```python
from build123d import *

# Parameters (mm, degrees)
F1_DEPTH    = 34.29
F2_T1_DEPTH = 186.4119082094
F2_T4_ANGLE = 180
F4_DEPTH    = 50.8
F6_DEPTH    = 27.94


# Not quite as in the source:
# - a fillet or chamfer that OpenCascade refuses, or shapes differently, is made with other operations: its cross-section is extruded or revolved along the edge and cut away or added


with BuildPart() as f1:
    # F0 (on Top) → F1 (new body)
    with BuildSketch(Plane.XY):
        with BuildLine():
            ThreePointArc((-39.772413671, 45.8196774125), (0, 6.0472637415), (39.772413671, 45.8196774125))
            Line((39.772413671, 45.8196774125), (-39.772413671, 45.8196774125))
        make_face()
        with BuildLine():
            Line((-39.772413671, 45.8196774125), (39.772413671, 45.8196774125))
            ThreePointArc((39.772413671, 45.8196774125), (0, 85.5920910835), (-39.772413671, 45.8196774125))
        make_face()
        with BuildLine():
            Line((39.772413671, -45.8196774125), (39.772413671, 45.8196774125))
            ThreePointArc((39.772413671, 45.8196774125), (0, 6.0472637415), (-39.772413671, 45.8196774125))
            Line((-39.772413671, 45.8196774125), (-39.772413671, -45.8196774125))
            Line((-39.772413671, -45.8196774125), (39.772413671, -45.8196774125))
        make_face()
    extrude(amount=F1_DEPTH)

    # F2: fillet of radius 38.1 on 3 edges, made by hand

    # F2_s2 → F2_t1 (cut)
    with BuildSketch(Plane.XZ.offset(-45.8196774125)):
        with BuildLine():
            ThreePointArc((-39.772413671, 0), (-27.4216493001, 24.4457162358), (-1.8633923173, 34.29))
            Line((-1.8633923173, 34.29), (-39.772413671, 34.29))
            Line((-39.772413671, 34.29), (-39.772413671, 0))
        make_face()
        with BuildLine():
            ThreePointArc((39.772413671, 0), (27.4216493001, 24.4457162358), (1.8633923173, 34.29))
            Line((1.8633923173, 34.29), (39.772413671, 34.29))
            Line((39.772413671, 34.29), (39.772413671, 0))
        make_face()
    extrude(amount=F2_T1_DEPTH, mode=Mode.SUBTRACT)

    # F2_s3 → F2_t4 (revolve, cut)
    with BuildSketch(Plane.XZ.offset(-45.8196774125)):
        with BuildLine():
            ThreePointArc((39.772413671, 0), (27.4216493001, 24.4457162358), (1.8633923173, 34.29))
            Line((1.8633923173, 34.29), (39.772413671, 34.29))
            Line((39.772413671, 34.29), (39.772413671, 0))
        make_face()
    revolve(axis=Axis((0, 45.8196774125, 34.29), (0, 0, 1)), revolution_arc=F2_T4_ANGLE, mode=Mode.SUBTRACT)

    # F3 (on Right) → F4 (cut)
    with BuildSketch(Plane.YZ):
        with BuildLine():
            add(Edge.make_bspline(
                [(26.3266563416, 13.0248842761), (26.3266563416, -3.7878693164), (55.981522426, 4.6185074799), (85.6363885105, 13.0248842761), (55.981522426, 21.4312610723), (26.3266563416, 29.8376378686), (26.3266563416, 13.0248842761)],
                knots=[0, 0, 0, 2.0943951024, 2.0943951024, 4.1887902048, 4.1887902048, 6.2831853072, 6.2831853072, 6.2831853072], degree=2, weights=[1, 0.5, 1, 0.5, 1, 0.5, 1]))
        make_face()
    extrude(amount=F4_DEPTH, mode=Mode.SUBTRACT)

    # F5 (on Right) → F6 (join)
    with BuildSketch(Plane.YZ):
        with BuildLine():
            add(Edge.make_bspline(
                [(65.8664852381, 13.2574718446), (65.8664852381, 30.580146327), (34.8160881549, 21.9188090858), (3.7656910717, 13.2574718446), (34.8160881549, 4.5961346033), (65.8664852381, -4.0652026379), (65.8664852381, 13.2574718446)],
                knots=[0, 0, 0, 2.0943951024, 2.0943951024, 4.1887902048, 4.1887902048, 6.2831853072, 6.2831853072, 6.2831853072], degree=2, weights=[1, 0.5, 1, 0.5, 1, 0.5, 1]))
        make_face()
    extrude(amount=F6_DEPTH)


solid = f1.part
```
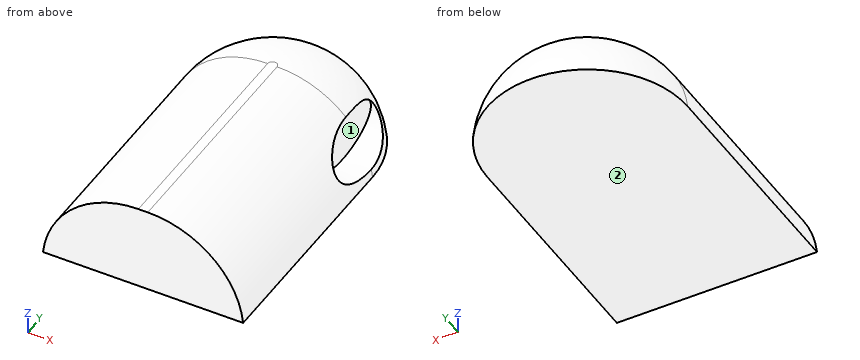
Check sheet for the modelled part. Datum: model origin and axes. Units: mm. Face numbers are marked on the shaded views. A direction names the side the tool comes from. Round coordinates to 2 decimals unless told otherwise and drop trailing zeros. Write each loop counter-clockwise with the first axis right and the second up, starting at its lowest first coordinate (ties: lowest second). Pieces come first, ordered by that corner, then holes. Notation, with made-up numbers: M -25.5,12 L -0.5,12 A11 ccw -0.5,23 Z; hole C -23,15.5 d5. An arc over 180 degrees is marked long. Write item = value, one per line. Start each with the question number.
1. Gauge pin test, flat ends, axial feed: pin 1 (2 mm diameter, centred on x = -22.5, y = -26, fed in from +Z); pin 2 (8 mm diameter, centred on y = -25.5, z = 15, fed in from +X); pin 3 (15.5 mm diameter, centred on y = 42, z = 11.5, fed in from +X); pin 4 (6 mm diameter, centred on x = -7.5, y = 4, fed in from -Z). Record the tip position at first contact, or that the pin passes through.
2. Section check A-A, the plane y = -27. Record the cut outline in (x, z), then the cut area to 3 significant figures.
3. Scan lines: line 1 (Z direction, x = -2, y = 45); line 2 (Y direction, x = 23.5, z = 8.5); line 3 (Y direction, x = 22.5, z = 7.5). Record each from-to range of solid material in increasing order. Write a range as [from, to].
4. Tool access check on the marked faces 1 and 2. Record the directions out of +Z, -Z, +X, -X, +Y, -Y that give a thin tool (end or side, any length) a straight path to the whole face; none if there is none.
Results found:
q1.pin_1 = 28.84
q1.pin_2 = 36.97
q1.pin_3 = 27.94
q1.pin_4 = 0
q2.outline = M -39.77,0 L 39.77,0 A38.1 ccw 1.86,34.29 L -1.86,34.29 A38.1 ccw Z
q2.area = 2,120 mm^2
q3.line_1 = [0, 34.29]
q3.line_2 = [-45.82, 63.37], [63.59, 75.58]
q3.line_3 = [-45.82, 62.09], [62.35, 76.75]
q4.face_1 = +X
q4.face_2 = -Z, +X, -X, +Y, -Y
